```python
from build123d import *

# Parameters (mm, degrees)
BOSS_EXTRUDE1_DEPTH = 30
SKETCH2_R           = 1.4
CUT_EXTRUDE1_DEPTH  = 90.675732638
SKETCH3_R           = 2.5
CUT_EXTRUDE2_DEPTH  = 1.5
CUT_EXTRUDE3_START  = -1.5
SKETCH4_R           = 2.5
CUT_EXTRUDE3_DEPTH  = 1.5
SKETCH5_R           = 11.4
CUT_EXTRUDE4_DEPTH  = 1.5
SKETCH6_R           = 3.1
SKETCH6_R_2         = 1
CUT_EXTRUDE5_DEPTH  = 57.184338839
FILLET1_R           = 5
FILLET2_R           = 2
SKETCH7_R           = 2.5
CUT_EXTRUDE6_DEPTH  = 1.5


with BuildPart() as part:
    # Sketch1 → Boss-Extrude1 (new body)
    with BuildSketch(Plane(origin=(0, 0, 0), x_dir=(1, 0, 0), z_dir=(0, 1, 0))):
        Polygon((65.823529412, -35.558823529), (65.823529412, -32.558823529), (37.323529412, -32.558823529), (37.323529412, 14.441176471), (65.823529412, 14.441176471), (65.823529412, 17.441176471), (32.823529412, 17.441176471), (32.823529412, -35.558823529), align=None)
    extrude(amount=BOSS_EXTRUDE1_DEPTH)

    # Sketch2 → Cut-Extrude1 (cut, through all)
    with BuildSketch(Plane(origin=(0, 0, -17.441176471), x_dir=(-1, 0, 0), z_dir=(0, 0, -1))):
        with Locations((-59.323529412, 9)):
            Circle(SKETCH2_R)
        with Locations((-43.323529412, 9)):
            Circle(SKETCH2_R)
        with Locations((-43.323529412, 21)):
            Circle(SKETCH2_R)
        with Locations((-59.323529412, 21)):
            Circle(SKETCH2_R)
    extrude(amount=-CUT_EXTRUDE1_DEPTH, mode=Mode.SUBTRACT)

    # Sketch3 → Cut-Extrude2 (cut)
    with BuildSketch(Plane(origin=(0, 0, -17.441176471), x_dir=(-1, 0, 0), z_dir=(0, 0, -1))):
        with Locations((-59.323529412, 9)):
            Circle(SKETCH3_R)
        with Locations((-43.323529412, 9)):
            Circle(SKETCH3_R)
        with Locations((-43.323529412, 21)):
            Circle(SKETCH3_R)
        with Locations((-59.323529412, 21)):
            Circle(SKETCH3_R)
    extrude(amount=-CUT_EXTRUDE2_DEPTH, mode=Mode.SUBTRACT)

    # Sketch4 → Cut-Extrude3 (cut)
    with BuildSketch(Plane.XY.offset(35.558823529).offset(CUT_EXTRUDE3_START)):
        with Locations(Location((59.323529412, 21, 0), (0, 0, 180))):
            Circle(SKETCH4_R)
        with Locations(Location((43.323529412, 21, 0), (0, 0, 180))):
            Circle(SKETCH4_R)
        with Locations(Location((43.323529412, 9, 0), (0, 0, 180))):
            Circle(SKETCH4_R)
        with Locations(Location((59.323529412, 9, 0), (0, 0, 180))):
            Circle(SKETCH4_R)
    extrude(amount=CUT_EXTRUDE3_DEPTH, mode=Mode.SUBTRACT)

    # Sketch5 → Cut-Extrude4 (cut)
    with BuildSketch(Plane.ZY.offset(-32.823529412)):
        with Locations((9.058823529, 15)):
            Circle(SKETCH5_R)
    extrude(amount=-CUT_EXTRUDE4_DEPTH, mode=Mode.SUBTRACT)

    # Sketch6 → Cut-Extrude5 (cut, through all)
    with BuildSketch(Plane.ZY.offset(-34.323529412)):
        with Locations((9.058823529, 15)):
            Circle(SKETCH6_R)
        with Locations((1.058823529, 15)):
            Circle(SKETCH6_R_2)
        with Locations((9.058823529, 23)):
            Circle(SKETCH6_R_2)
        with Locations((17.058823529, 15)):
            Circle(SKETCH6_R_2)
        with Locations((9.058823529, 7)):
            Circle(SKETCH6_R_2)
    extrude(amount=-CUT_EXTRUDE5_DEPTH, mode=Mode.SUBTRACT)

    # Fillet1
    fillet1_edges = [part.edges().sort_by_distance(p)[0] for p in [
        (65.823529412, 0, 34.058823529),
        (65.823529412, 30, -15.941176471),
        (65.823529412, 30, 34.058823529),
        (65.823529412, 0, -15.941176471),
    ]]
    fillet(fillet1_edges, radius=FILLET1_R)

    # Fillet2
    fillet2_edges = [part.edges().sort_by_distance(p)[0] for p in [
        (32.823529412, 15, 35.558823529),
        (32.823529412, 15, -17.441176471),
    ]]
    fillet(fillet2_edges, radius=FILLET2_R)

    # Sketch7 → Cut-Extrude6 (cut)
    with BuildSketch(Plane(origin=(37.323529412, 0, 0), x_dir=(0, 0, -1), z_dir=(1, 0, 0))):
        with Locations((-17.058823529, 15)):
            Circle(SKETCH7_R)
        with Locations((-9.058823529, 23)):
            Circle(SKETCH7_R)
        with Locations((-1.058823529, 15)):
            Circle(SKETCH7_R)
        with Locations((-9.058823529, 7)):
            Circle(SKETCH7_R)
    extrude(amount=-CUT_EXTRUDE6_DEPTH, mode=Mode.SUBTRACT)


solid = part.part
```
Geometry: final body of the model. Coordinates: model frame, mm. A direction names the side the tool comes from. Round coordinates to 2 decimals unless told otherwise and drop trailing zeros. Write each loop counter-clockwise with the first axis right and the second up, starting at its lowest first coordinate (ties: lowest second). Pieces come first, ordered by that corner, then holes.
Item 1: Section query C-C (y = 27.75). Return loops of the section in (x, z), plus the area to 3 significant figures.
Item 2: Material intervals for L1, parallel to Z at x = 38, y = 6.5; L2, parallel to Z at x = 42.5, y = 11; L3, parallel to X at y = 21, z = 34.6, sorted ascending.
Item 3: Set-up query: faces 3 (the face through (59.87, 11.44, 34.8)), 4 (the face through (58, 8, -15.941)), 5 (the face through (36.58, 6.04, 6.75)). Return all of +Z, -Z, +X, -X, +Y, -Y with unobstructed straight access to the full face (end or side cutting, diameter ignored); none if empty.
Item 4: Section query B-B (y = 15). Give the number of separate pieces and of enclosed holes in the cut face, plus the area to 3 significant figures.
Item 5: Section query D-D (z = -4). Return loops of the section in (x, y), plus the area to 3 significant figures.
Item 6: Section query A-A (x = 51). Return loops of the section in (y, z), plus the area to 3 significant figures.
Item 7: Pin query (flat end, axial travel): P1, Ø8, axis at y = 15, z = 17.06, coming from the +X side; P2, Ø2.5, axis at x = 43.5, y = 10, coming from the +Z side; P3, Ø1.2, axis at y = 23, z = 9.06, coming from the +X side; P4, Ø2.5, axis at y = 15.5, z = 18, coming from the +X side. Return the tip coordinate at first contact, or that it passes through.
Item 8: Mould query, pull axis Y, two halves, no side actions, for faces 1 (the face through (52, 15, 32.559)), 2 (the face through (42, 10, 34.059)). Classes: +Y half, -Y half, draft (parallel to the pull), parting line (faces both ways), or undercut.
Completed:
1. outline: (32.82, -15.44) arc R2 ccw to (34.82, -17.44) - (65, -17.44) - (65, -14.44) - (37.32, -14.44) - (37.32, 32.56) - (65, 32.56) - (65, 35.56) - (34.82, 35.56) arc R2 ccw to (32.82, 33.56) - close
1. area: 403 mm2
2. L1: z = -17.44 to -14.44, 32.56 to 35.56
2. L2: z = -15.94 to -14.44, 32.56 to 34.06
2. L3: x = 33.12 to 40.82, 45.82 to 56.82, 61.82 to 65.82
3. face 3: +Z
3. face 4: -Z
3. face 5: +X
4. separate pieces: 4
4. enclosed holes: 0
4. area: 334 mm2
5. outline: (32.82, 0) - (37.32, 0) - (37.32, 30) - (32.82, 30) - close
5. area: 135 mm2
6. outline: (0, -17.44) - (30, -17.44) - (30, -14.44) - (0, -14.44) - close; (0, 32.56) - (30, 32.56) - (30, 35.56) - (0, 35.56) - close
6. area: 180 mm2
7. P1: stops at x = 37.32
7. P2: stops at z = 34.06
7. P3: passes through
7. P4: stops at x = 35.82
8. face 1: draft
8. face 2: undercut
